Work out the finished part from the listing and answer in its coordinate system (mm). Coordinates: 2 decimals unless noted, no trailing zeros. Order: outer loops, then holes, each group sorted by start corner. A loop starts at its lowest first (then second) coordinate and runs counter-clockwise, first axis right, second up.
```python
from build123d import *

# Parameters (mm, degrees)
BOSS_EXTRUDE1_DEPTH = 2.5
SKETCH4_R           = 0.375
BOSS_EXTRUDE3_DEPTH = 8
LPATTERN1_COUNT     = 2
LPATTERN1_PITCH     = 38.1


with BuildPart() as part:
    # Sketch2 → Boss-Extrude1 (new body)
    with BuildSketch(Plane(origin=(0, 0, 0), x_dir=(1, 0, 0), z_dir=(0, 1, 0))):
        with BuildLine():
            Line((-4, 22), (4, 22))
            ThreePointArc((4, 22), (6.121320344, 21.121320344), (7, 19))
            Line((7, 19), (7, -19))
            ThreePointArc((7, -19), (6.121320344, -21.121320344), (4, -22))
            Line((4, -22), (-4, -22))
            ThreePointArc((-4, -22), (-6.121320344, -21.121320344), (-7, -19))
            Line((-7, -19), (-7, 19))
            ThreePointArc((-7, 19), (-6.121320344, 21.121320344), (-4, 22))
        make_face()
    extrude(amount=BOSS_EXTRUDE1_DEPTH)

    # Sketch4 → Boss-Extrude3 (add)
    with BuildSketch(Plane.XZ):
        with Locations(Location((-5, 19.46, 0), (0, 0, 90))):
            Circle(SKETCH4_R)
        with Locations(Location((-1.67, 19.46, 0), (0, 0, 90))):
            Circle(SKETCH4_R)
        with Locations(Location((1.66, 19.46, 0), (0, 0, 90))):
            Circle(SKETCH4_R)
        with Locations(Location((4.99, 19.46, 0), (0, 0, 90))):
            Circle(SKETCH4_R)
    boss_extrude3 = extrude(amount=BOSS_EXTRUDE3_DEPTH)

    # LPattern1: Boss-Extrude3 ×2
    with Locations(*[(0, 0, -i * LPATTERN1_PITCH) for i in range(1, LPATTERN1_COUNT)]):
        add(boss_extrude3)


solid = part.part
```
1. The part is cut by section C-C (z = 15). Determine the outline of the cut face in (x, y).
2. Consider probe 1 along Z at (x, y) = (-5, -4.5) (3 decimals); probe 2 along Y at (x, z) = (-0.5, 14); probe 3 along Z at (x, y) = (5.25, -2). Determine where each line is inside the solid, lowest interval first.
3. The part is cut by section B-B (x = -0.5). Determine the outline of the cut face in (y, z), plus the area to 3 significant figures.
4. Flat-ended cylindrical pins translate along their axes: pin 1 (1 mm diameter, centred on x = -4, y = -4.5, fed in from +Z); pin 2 (7 mm diameter, centred on x = -1.5, z = 10, fed in from -Y); pin 3 (1.5 mm diameter, centred on x = -5.5, y = -6.5, fed in from +Z) (3 decimals). Find the tip coordinate at first contact, or state that the pin passes through.
5. The part is cut by section A-A (y = -7.25). Determine the outline of the cut face in (x, z) (3 decimals).
Worked out:
1. outline: (-7, 0) - (7, 0) - (7, 2.5) - (-7, 2.5) - close
2. probe 1: z = -19.015 to -18.265, 19.085 to 19.835
2. probe 2: y = 0 to 2.5
2. probe 3: z = -18.91 to -18.37, 19.19 to 19.73
3. outline: (0, -22) - (2.5, -22) - (2.5, 22) - (0, 22) - close
3. area: 110 mm2
4. pin 1: passes through
4. pin 2: stops at y = 0
4. pin 3: stops at z = 19.835
5. outline: circle Ø0.75 at (-5, -18.64); circle Ø0.75 at (-5, 19.46); circle Ø0.75 at (-1.67, -18.64); circle Ø0.75 at (-1.67, 19.46); circle Ø0.75 at (1.66, -18.64); circle Ø0.75 at (1.66, 19.46); circle Ø0.75 at (4.99, -18.64); circle Ø0.75 at (4.99, 19.46)
